Input: part model. Units: mm. Frame: model coordinates. Face numbers are marked on the shaded views. Coordinates: 2 decimals unless noted, no trailing zeros. Order: outer loops, then holes, each group sorted by start corner. A loop starts at its lowest first (then second) coordinate and runs counter-clockwise, first axis right, second up. Notation, with made-up numbers: (40.25, 37.25) -> (72.25, 37.25) arc R25 cw to (72.25, 54.25) -> close; hole circle Ø9 at (21.25, -27.75). An arc over 180 degrees is marked (long way). One line per question, with ' | ' between items.
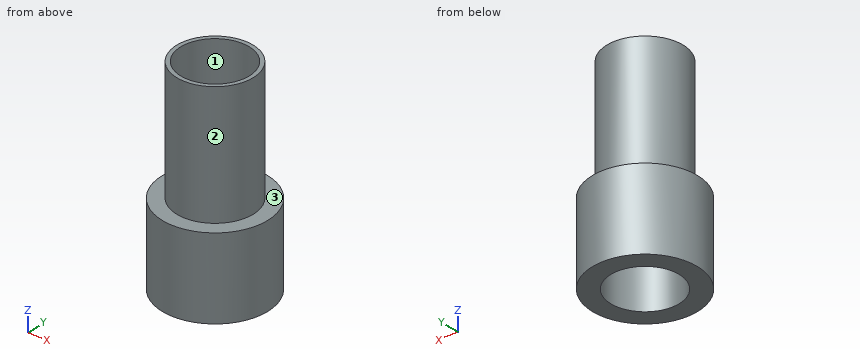
```python
from build123d import *

# Parameters (mm, degrees)
F0_R     = 41.275
F1_DEPTH = 158.75
F2_R     = 41.275
F2_R_2   = 29.972
F3_DEPTH = 95.25
F4_R     = 26.8605
F5_DEPTH = 158.751


with BuildPart() as f1:
    # F0 (on Top) → F1 (new body)
    with BuildSketch(Plane.XY):
        Circle(F0_R)
    extrude(amount=F1_DEPTH)

    # F2 (on face) → F3 (cut)
    with BuildSketch(Plane.XY.offset(158.75)):
        Circle(F2_R)
        Circle(F2_R_2, mode=Mode.SUBTRACT)
    extrude(amount=-F3_DEPTH, mode=Mode.SUBTRACT)

    # F4 (on face) → F5 (cut, through all)
    with BuildSketch(Plane.XY.offset(158.75)):
        Circle(F4_R)
    extrude(amount=-F5_DEPTH, mode=Mode.SUBTRACT)


solid = f1.part
```
1. Ray query, line 1 (Y direction, x = 0, z = 43.5) (1 decimal); line 2 (Z direction, x = 33, y = -17); line 3 (X direction, y = 15.5, z = 17.5). Return the intervals inside material, ascending. Write a range as [from, to].
Recorded:
line 1: y = [-41.3, -26.9], [26.9, 41.3] | line 2: z = [0, 63.5] | line 3: x = [-38.25, -21.94], [21.94, 38.25]
2. Pin query (flat end, axial travel): pin 1 Ø1 at (x, z) = (22, 141) entering from -Y; pin 2 Ø1.5 at (x, z) = (-22, 64) entering from -Y; pin 3 Ø3 at (y, z) = (28.5, 120.5) entering from +X. Return the tip coordinate at first contact, or that it passes through.
Recorded:
pin 1: stops at y = -20.88 | pin 2: stops at y = -35.27 | pin 3: stops at x = 13.01
3. Mould query, pull axis X, two halves, no side actions, for the marked faces 1, 2 and 3. Classes: released by +X, released by -X, zero draft, split by the parting line, or undercut.
Recorded:
face 1: undercut | face 2: split by the parting line | face 3: zero draft
4. Cut plane C-C, the plane z = 122. Return loops of the section in (x, y).
Recorded:
outline: circle Ø59.94 at (0, 0); hole circle Ø53.72 at (0, 0)
